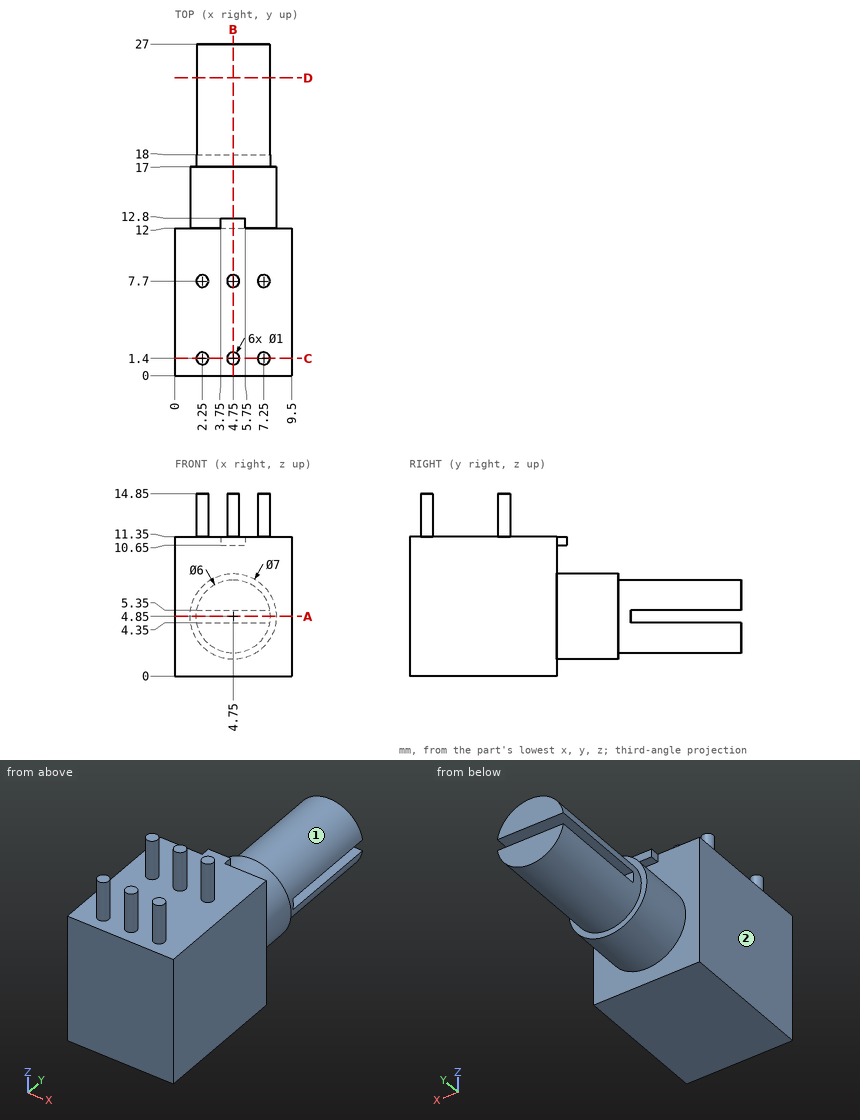
Can you work these out from the drawing? Everything is in mm from the part's minimum corner. A direction names the side the tool comes from. Give positions to 0.01 mm unless a question says otherwise; leave off trailing zeros. Loops run counter-clockwise (first coordinate to the right, second up) from the corner with the lowest first, then second, coordinate; pieces in that order, holes last. Notation, with made-up numbers: M 39,65 L 48,65 A17 cw 48,88 Z; hole C 86.5,70 d10. An arc over 180 degrees is marked long. Use CSV: the item, a comma, the result in double quotes. Start each with the question number.
1. On a 3-axis mill with a long thin cutter (end or side, diameter ignored), from which of +Z, -Z, +X, -X, +Y, -Y can I reach the whole of each face in a straight line? I mean the marked faces 1 and 2. Say none if no direction works.
2. For P1, Ø4, axis at y = 8.5, z = 9.5, coming from the -X side; P2, Ø1.5, axis at x = 1.5, y = 6.5, coming from the +Z side; P3, Ø4.5, axis at x = 5.5, y = 22.5, coming from the -Z side; P4, Ø3, axis at x = 4, y = 22, coming from the +Z side, each with a flat end and sliding along its axis, tell me the tip position at first contact or that it passes through.
3. If I drill on L1, parallel to Z at x = 4.75, y = 11.25; L2, parallel to Z at x = 5, y = 22.75; L3, parallel to Y at x = 8.5, z = 9.5, over which ranges is the centre line in solid material (lowest first)?
4. Imagine slicing it at B-B, the plane x = 4.75. Write out the boundary of the cut face in (y, z), plus the area to 3 significant figures.
5. Imagine slicing it at A-A, the plane z = 4.85. Write out the boundary of the cut face in (x, y), plus the area to 3 significant figures.
6. Imagine slicing it at D-D, the plane y = 24.25. Write out the boundary of the cut face in (x, z).
7. Imagine slicing it at C-C, the plane y = 1.4. Write out the boundary of the cut face in (x, z), plus the area to 3 significant figures.
Response values:
1,face 1,"+Y"
1,face 2,"+Z, -Z, -X, +Y, -Y"
2,P1,"x = 0"
2,P2,"z = 11.35"
2,P3,"z = 1.85"
2,P4,"z = 7.85"
3,L1,"0 to 11.35"
3,L2,"1.86 to 4.35, 5.35 to 7.84"
3,L3,"0 to 12"
4,outline,"M 0,0 L 12,0 L 12,1.35 L 17,1.35 L 17,1.85 L 27,1.85 L 27,4.35 L 18,4.35 L 18,5.35 L 27,5.35 L 27,7.85 L 17,7.85 L 17,8.35 L 12,8.35 L 12,10.65 L 12.8,10.65 L 12.8,11.35 L 8.2,11.35 L 8.2,14.85 L 7.2,14.85 L 7.2,11.35 L 1.9,11.35 L 1.9,14.85 L 0.9,14.85 L 0.9,11.35 L 0,11.35 Z"
4,area,"230 mm^2"
5,outline,"M 0,0 L 9.5,0 L 9.5,12 L 8.25,12 L 8.25,17 L 7.75,17 L 7.75,18 L 1.75,18 L 1.75,17 L 1.25,17 L 1.25,12 L 0,12 Z"
5,area,"155 mm^2"
6,outline,"M 1.79,4.35 A3 ccw 7.71,4.35 Z; M 1.79,5.35 L 7.71,5.35 A3 ccw Z"
7,outline,"M 0,0 L 9.5,0 L 9.5,11.35 L 7.75,11.35 L 7.75,14.85 L 6.75,14.85 L 6.75,11.35 L 5.25,11.35 L 5.25,14.85 L 4.25,14.85 L 4.25,11.35 L 2.75,11.35 L 2.75,14.85 L 1.75,14.85 L 1.75,11.35 L 0,11.35 Z"
7,area,"118 mm^2"
